The figure shows three views and two pictorial views of one solid part (mm, origin at its lowest corner). Answer the questions. A direction names the side the tool comes from. Give positions to 0.01 mm unless a question says otherwise; leave off trailing zeros. Write each loop counter-clockwise with the first axis right and the second up, starting at its lowest first coordinate (ties: lowest second). Pieces come first, ordered by that corner, then holes. Notation, with made-up numbers: (7.25, -3.5) -> (50.25, -3.5) arc R22 ccw to (50.25, 25.5) -> close; hole circle Ø11 at (6.25, -38.75). An arc over 180 degrees is marked (long way). Use a Markdown table: item, result.
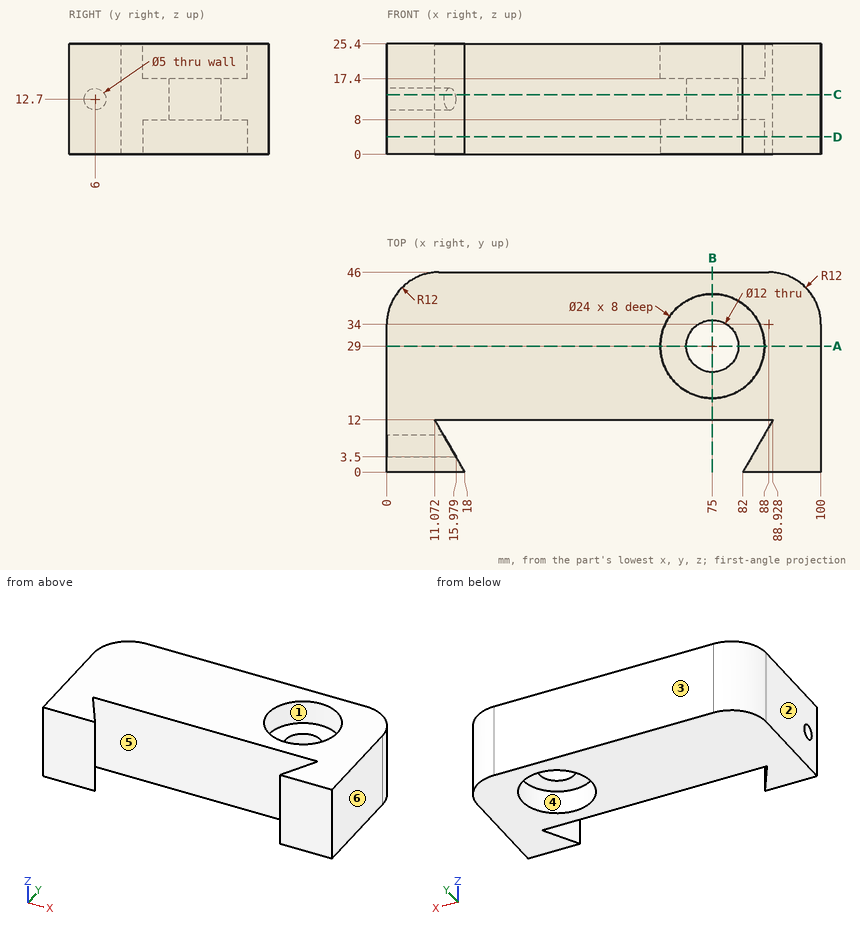
Item 1: A tool of negligible diameter and unlimited length cuts with its end or side. For the marked faces 5 and 6, from which of +Z, -Z, +X, -X, +Y, -Y can it reach the whole face along a straight path? Write none if from no direction.
Return value:
| item | result |
|---|---|
| face 5 | +Z, -Z |
| face 6 | +Z, -Z, +X, +Y, -Y |
Item 2: A cutting plane is placed at A-A (y = 29). Give the vertices of the cut face in (x, z), then the cut area to 3 significant figures.
Return value:
| item | result |
|---|---|
| outline | (0, 0) -> (63, 0) -> (63, 8) -> (69, 8) -> (69, 17.4) -> (63, 17.4) -> (63, 25.4) -> (0, 25.4) -> close; (81, 8) -> (87, 8) -> (87, 0) -> (100, 0) -> (100, 25.4) -> (87, 25.4) -> (87, 17.4) -> (81, 17.4) -> close |
| area | 2,040 mm^2 |
Item 3: Each of these flat-tipped pins is pushed along its axis until it touches: P1, Ø4, axis at y = 6, z = 12.7, coming from the -X side; P2, Ø14.5, axis at x = 75, y = 29, coming from the +Z side; P3, Ø4, axis at x = 36, z = 10, coming from the -Y side. Where does it stop, or does it pass through?
Return value:
| item | result |
|---|---|
| P1 | x = 84.31 |
| P2 | z = 17.4 |
| P3 | y = 12 |
Item 4: A cutting plane is placed at C-C (z = 13.75). Give the vertices of the cut face in (x, y).
Return value:
| item | result |
|---|---|
| outline | (0, 0) -> (18, 0) -> (15.85, 3.73) -> (0, 3.73) -> close; (0, 8.27) -> (13.23, 8.27) -> (11.07, 12) -> (88.93, 12) -> (82, 0) -> (100, 0) -> (100, 34) arc R12 ccw to (88, 46) -> (12, 46) arc R12 ccw to (0, 34) -> close; hole circle Ø12 at (75, 29) |
Item 5: A cutting plane is placed at B-B (x = 75). Give the vertices of the cut face in (y, z).
Return value:
| item | result |
|---|---|
| outline | (12, 0) -> (17, 0) -> (17, 8) -> (23, 8) -> (23, 17.4) -> (17, 17.4) -> (17, 25.4) -> (12, 25.4) -> close; (35, 8) -> (41, 8) -> (41, 0) -> (46, 0) -> (46, 25.4) -> (41, 25.4) -> (41, 17.4) -> (35, 17.4) -> close |
Item 6: For a pull along Y with two mould halves and no side action, classify the marked faces 1, 2, 3 and 4 as +Y half, -Y half, draft (parallel to the pull), parting line (faces both ways), or undercut.
Return value:
| item | result |
|---|---|
| face 1 | undercut |
| face 2 | draft |
| face 3 | +Y half |
| face 4 | undercut |
Item 7: A cutting plane is placed at D-D (z = 4). Give the vertices of the cut face in (x, y).
Return value:
| item | result |
|---|---|
| outline | (0, 0) -> (18, 0) -> (11.07, 12) -> (88.93, 12) -> (82, 0) -> (100, 0) -> (100, 34) arc R12 ccw to (88, 46) -> (12, 46) arc R12 ccw to (0, 34) -> close; hole circle Ø24 at (75, 29) |
Item 8: Straight lines are drawn through the part: line 1 along X through (y, z) = (29, 10.5); line 2 along Y through (x, z) = (75, 3.25); line 3 along Z through (x, y) = (12.5, 6). For each, find the intervals that lie inside material, in ascending order. Write a range as [from, to].
Return value:
| item | result |
|---|---|
| line 1 | [0, 69], [81, 100] |
| line 2 | [12, 17], [41, 46] |
| line 3 | [0, 10.2], [15.2, 25.4] |
